```python
from build123d import *

# Parameters (mm, degrees)
SKETCH_3_R      = 1.7
EXTRUDE_3_DEPTH = 4
CHAMFER_1_SIZE  = 30
FILLET_1_R      = 3


with BuildPart() as part:
    # 草图3 → 凸台-拉伸3 (new body)
    with BuildSketch(Plane(origin=(0, 0, 0), x_dir=(0, 0, -1), z_dir=(1, 0, 0))):
        Polygon((0, 0), (80, 0), (90, 0), (90, 80), (80, 80), align=None)
        with Locations((85, 5)):
            Circle(SKETCH_3_R, mode=Mode.SUBTRACT)
        with Locations((85, 70)):
            Circle(SKETCH_3_R, mode=Mode.SUBTRACT)
        with Locations((62.32233047, 55.251262658)):
            Circle(SKETCH_3_R, mode=Mode.SUBTRACT)
        with Locations((34.038059223, 26.966991411)):
            Circle(SKETCH_3_R, mode=Mode.SUBTRACT)
    extrude(amount=EXTRUDE_3_DEPTH)

    # 倒角1
    chamfer_1_edges = [part.edges().sort_by_distance(p)[0] for p in [
        (2, 0, 0),
    ]]
    chamfer(chamfer_1_edges, length=CHAMFER_1_SIZE)

    # 圆角1
    fillet_1_edges = [part.edges().sort_by_distance(p)[0] for p in [
        (2, 0, -30),
        (2, 21.213203436, -21.213203436),
        (2, 80, -80),
        (2, 80, -90),
        (2, 0, -90),
    ]]
    fillet(fillet_1_edges, radius=FILLET_1_R)


solid = part.part
```
Here's how the part is built. I have some questions about the finished solid (model axes, mm). Give positions to 0.01 mm unless a question says otherwise; leave off trailing zeros. Order: outer loops, then holes, each group sorted by start corner. A loop starts at its lowest first (then second) coordinate and runs counter-clockwise, first axis right, second up. Notation, with made-up numbers: (-31.75, -19) -> (-19.75, -19) arc R17 ccw to (-19.75, -10) -> close; hole circle Ø8 at (83, 64.5). An arc over 180 degrees is marked (long way). Use CSV: the item, a comma, the result in double quotes. Start each with the question number.
Item 1: Suppose I cut it at A-A (y = 70). List the corners of the cut face in (x, z) for me.
Item 2: I'm going to push flat-ended pins straight in: P1, Ø2, axis at x = 2.5, y = 48.5, coming from the +Z side; P2, Ø3, axis at y = 26.97, z = -34.04, coming from the -X side. Where does each tip first touch, or does it pass through?
Item 3: Suppose I cut it at B-B (z = -85). List the corners of the cut face in (x, y) for me, and give its area (3 significant figures).
Item 4: Thinking about a two-plate mould opening in Y: for faces 1 (the flat face through (2, 51, -51)), 2 (the flat face through (0, 32, -63)), 3 (the cylindrical face through (1.97, 5.07, -83.3)), which applies, pulls with the +Y half, pulls with the -Y half, needs draft (parallel to the pull), parting line crosses it, or undercut?
Item 5: Suppose I cut it at D-D (z = -45.5). List the corners of the cut face in (x, y) for me.
Item 6: If I drill on probe 1 along Y at (x, z) = (2.35, -85); probe 2 along Z at (x, y) = (1.7, 32); probe 3 along Z at (x, y) = (1.4, 6), over which ranges is the centre line in solid material (lowest first)? Write a range as [from, to].
Item 7: Suppose I cut it at C-C (x = 1.4). List the corners of the cut face in (y, z) for me, and give its area (3 significant figures).
Answer block:
1,outline,"(0, -90) -> (4, -90) -> (4, -86.7) -> (0, -86.7) -> close; (0, -83.3) -> (4, -83.3) -> (4, -70) -> (0, -70) -> close"
2,P1,"stops at z = -47.5"
2,P2,"passes through"
3,outline,"(0, 0) -> (4, 0) -> (4, 3.3) -> (0, 3.3) -> close; (0, 6.7) -> (4, 6.7) -> (4, 68.3) -> (0, 68.3) -> close; (0, 71.7) -> (4, 71.7) -> (4, 80) -> (0, 80) -> close"
3,area,"293 mm^2"
4,face 1,"pulls with the +Y half"
4,face 2,"needs draft"
4,face 3,"undercut"
5,outline,"(0, 0) -> (4, 0) -> (4, 45.5) -> (0, 45.5) -> close"
6,probe 1,"y = [0, 3.3], [6.7, 68.3], [71.7, 80]"
6,probe 2,"z = [-90, -32]"
6,probe 3,"z = [-90, -86.37], [-83.63, -27.51]"
7,outline,"(0, -87) arc R3 ccw to (3, -90) -> (77, -90) arc R3 ccw to (80, -87) -> (80, -81.24) arc R3 ccw to (79.12, -79.12) -> (22.63, -22.63) arc R3 ccw to (19.36, -21.98) -> (1.85, -29.23) arc R3 ccw to (0, -32) -> close; hole circle Ø3.4 at (5, -85); hole circle Ø3.4 at (26.97, -34.04); hole circle Ø3.4 at (55.25, -62.32); hole circle Ø3.4 at (70, -85)"
7,area,"3,640 mm^2"
